Model file for the job. Use its own axes, mm. A direction names the side the tool comes from. Give positions to 0.01 mm unless a question says otherwise; leave off trailing zeros. Order: outer loops, then holes, each group sorted by start corner. A loop starts at its lowest first (then second) coordinate and runs counter-clockwise, first axis right, second up. Notation, with made-up numbers: (-16, 28.5) -> (36, 28.5) arc R24 cw to (36, 59.5) -> close; hole circle Ø2 at (80.25, -5.5). An arc over 180 degrees is marked (long way). Answer in a Markdown table with one row per item. Add a question column.
from build123d import *

# Parameters (mm, degrees)
BOSS_EXTRUDE1_DEPTH = 12.7
SKETCH3_R           = 1.27
CUT_EXTRUDE1_DEPTH  = 12.7
CUT_EXTRUDE2_DEPTH  = 3.937
LPATTERN1_COUNT     = 3
LPATTERN1_PITCH     = 31.75
CUT_EXTRUDE3_DEPTH  = 2.54


with BuildPart() as part:
    # Sketch2 → Boss-Extrude1 (new body)
    with BuildSketch(Plane.XY):
        with BuildLine():
            Line((0, 0), (38.1, 0))
            Line((38.1, 0), (38.1, 8.255))
            Line((38.1, 8.255), (22.86, 8.255))
            ThreePointArc((22.86, 8.255), (36.352714712, 32.797844463), (28.528615071, 59.69))
            Line((28.528615071, 59.69), (22.910736376, 59.69))
            ThreePointArc((22.910736376, 59.69), (-0.00316084, 4.419599864), (-22.917058056, 59.69))
            Line((-22.917058056, 59.69), (-28.534936751, 59.69))
            ThreePointArc((-28.534936751, 59.69), (-36.359036392, 32.797844463), (-22.86632168, 8.255))
            Line((-22.86632168, 8.255), (-38.1, 8.255))
            Line((-38.1, 8.255), (-38.1, 0))
            Line((-38.1, 0), (0, 0))
        make_face()
    extrude(amount=BOSS_EXTRUDE1_DEPTH)

    # Sketch3 → Cut-Extrude1 (cut)
    with BuildSketch(Plane.XZ):
        with Locations(Location((0, 6.35, 0), (0, 0, 270))):
            Circle(SKETCH3_R)
        with Locations(Location((31.75, 6.35, 0), (0, 0, 270))):
            Circle(SKETCH3_R)
        with Locations(Location((-31.75, 6.35, 0), (0, 0, 270))):
            Circle(SKETCH3_R)
    extrude(amount=-CUT_EXTRUDE1_DEPTH, mode=Mode.SUBTRACT)

    # Sketch4 → Cut-Extrude2 (cut)
    with BuildSketch(Plane(origin=(0, 8.255, 0), x_dir=(1, 0, 0), z_dir=(0, 1, 0))):
        Polygon((-30.415911199, -8.690045044), (-33.129332156, -8.690045044), (-34.502956004, -6.35), (-33.28343783, -3.926071637), (-30.570033405, -3.91660003), (-29.20512854, -6.26174139), align=None)
    cut_extrude2 = extrude(amount=-CUT_EXTRUDE2_DEPTH, mode=Mode.SUBTRACT)

    # LPattern1: Cut-Extrude2 ×3
    with Locations(*[(i * LPATTERN1_PITCH, 0, 0) for i in range(1, LPATTERN1_COUNT)]):
        add(cut_extrude2, mode=Mode.SUBTRACT)

    # Sketch6 → Cut-Extrude3 (cut)
    with BuildSketch(Plane(origin=(0, 4.318, 0), x_dir=(1, 0, 0), z_dir=(0, 1, 0))):
        Polygon((1.334088801, -8.690045044), (-1.379332156, -8.690045044), (-2.752956004, -6.35), (-1.53343783, -3.926071637), (1.179966595, -3.91660003), (2.54487146, -6.26174139), align=None)
    extrude(amount=-CUT_EXTRUDE3_DEPTH, mode=Mode.SUBTRACT)


solid = part.part
Item 1: Wall check: line 1 (X direction, y = 1.65, z = 6.35); line 2 (X direction, y = 3.3, z = 6.35); line 3 (Y direction, x = -29, z = 1) (3 decimals). Give the ranges that are in metal, low to high.
Item 2: Saw through at C-C on z = 3. List the corners of the cut face in (x, y) (3 decimals).
Item 3: Saw through at B-B on x = 0. List the corners of the cut face in (y, z), plus the area to 3 significant figures.
Item 4: Pin check, flat tips, straight feed: pin 1 Ø2.5 at (x, z) = (-31, 6) entering from +Y; pin 2 Ø2.5 at (x, z) = (-0.5, 5.5) entering from +Y; pin 3 Ø4 at (x, z) = (-31, 6.5) entering from +Y; pin 4 Ø1 at (x, y) = (2, 6) entering from +Z. Stop position of each tip, or through.
Item 5: Saw through at A-A on y = 13.5. List the corners of the cut face in (x, z).
Item 6: Two-plate mould, pull along Y, no slides. Class faces 4 (the flat face through (33.6, 6.31, 5.07)), 5 (the flat face through (-1, 0, 8)), 6 (the flat face through (0, 3, 8.69)): pulls with the +Y half, pulls with the -Y half, needs draft (parallel to the pull), parting line crosses it, or undercut.
Item 7: Which spindle directions (+Z, -Z, +X, -X, +Y, -Y) get a long thin tool onto all of the face, cutting with end or side? Do faces 1 (the cylindrical face through (30.51, 2.13, 6.63)), 2 (the flat face through (-29.802, 6.314, 7.459)), 3 (the flat face through (1.948, 3.168, 7.459)). Say none if no direction does.
Item 8: Saw through at D-D on y = 50. List the corners of the cut face in (x, z).
Evaluation:
| question | item | result |
|---|---|---|
| 1 | line 1 | x = -38.1 to -33.02, -30.48 to -1.27, 1.27 to 30.48, 33.02 to 38.1 |
| 1 | line 2 | x = -38.1 to -33.02, -30.48 to -2.75, 2.5 to 30.48, 33.02 to 38.1 |
| 1 | line 3 | y = 0 to 8.255, 14.511 to 22.383, 51.226 to 59.098 |
| 2 | outline | (-38.1, 0) -> (38.1, 0) -> (38.1, 8.255) -> (22.86, 8.255) arc R36.576 ccw to (28.529, 59.69) -> (22.911, 59.69) arc R32.385 cw (long way) to (-22.917, 59.69) -> (-28.535, 59.69) arc R36.576 ccw to (-22.866, 8.255) -> (-38.1, 8.255) -> close |
| 3 | outline | (0, 0) -> (4.42, 0) -> (4.42, 3.92) -> (1.78, 3.92) -> (1.78, 5.08) -> (0, 5.08) -> close; (0, 7.62) -> (1.78, 7.62) -> (1.78, 8.69) -> (4.42, 8.69) -> (4.42, 12.7) -> (0, 12.7) -> close |
| 3 | area | 39.0 mm2 |
| 4 | pin 1 | stops at y = 58.09 |
| 4 | pin 2 | stops at y = 1.78 |
| 4 | pin 3 | stops at y = 59.1 |
| 4 | pin 4 | passes through |
| 5 | outline | (-28.19, 0) -> (-22.49, 0) -> (-22.49, 12.7) -> (-28.19, 12.7) -> close; (22.48, 0) -> (28.19, 0) -> (28.19, 12.7) -> (22.48, 12.7) -> close |
| 6 | face 4 | undercut |
| 6 | face 5 | pulls with the -Y half |
| 6 | face 6 | needs draft |
| 7 | face 1 | -Y |
| 7 | face 2 | none |
| 7 | face 3 | +Y |
| 8 | outline | (-34.12, 0) -> (-29.58, 0) -> (-29.58, 12.7) -> (-34.12, 12.7) -> close; (29.57, 0) -> (34.11, 0) -> (34.11, 12.7) -> (29.57, 12.7) -> close |
